The model under review builds one solid part; all positions refer to its coordinate system, in mm. A direction names the side the tool comes from. Round coordinates to 2 decimals unless told otherwise and drop trailing zeros. Loops run counter-clockwise (first coordinate to the right, second up) from the corner with the lowest first, then second, coordinate; pieces in that order, holes last. Notation, with made-up numbers: (-9.75, -24.5) -> (25.25, -24.5) arc R27 cw to (25.25, -4.5) -> close; hole circle Ø5 at (64.25, -29.5). An arc over 180 degrees is marked (long way). Write each question's results on one line, items separated by ' | '. Start each with the question number.
Item 1: For L1, parallel to Y at x = 33, z = -48; L2, parallel to Y at x = 40.5, z = -73; L3, parallel to X at y = 20, z = -83.5, list the stretches that pass through material, from the lowest coordinate up. Write a range as from..to.
Item 2: We need section C-C (z = -68.5). Give the boundary of the cut face in (x, y), and give its area (3 significant figures).
Item 3: Clearance check with flat-ended pins moving along their axes: pin 1 Ø10 at (y, z) = (22, -77.5) entering from +X; pin 2 Ø12 at (x, z) = (39, -17.5) entering from +Y; pin 3 Ø12 at (y, z) = (28.5, -60) entering from +X. State where each tip first meets the part, or that it passes through.
Item 4: We need section D-D (x = 47). Give the boundary of the cut face in (y, z), and give its area (3 significant figures).
Item 5: Tool access review of faces 1 (the cylindrical face through (25.819, 18.961, -50.805)), 2 (the flat face through (26, 0, -44)), 3 (the flat face through (44.45, 19, -80)), 4 (the cylindrical face through (15.322, 31.661, -77.578)), 5 (the flat face through (6.35, 19, -79)): name each direction out of +Z, -Z, +X, -X, +Y, -Y from which nothing blocks a thin tool from reaching the whole face with its end or side.
Item 6: We need section A-A (x = 25.4). Give the boundary of the cut face in (y, z), and give its area (3 significant figures).
Item 7: We need section B-B (y = 28.5). Give the boundary of the cut face in (x, z).
Autodesk Inventor part; units mm, degrees
ref_plane "YZ Plane" through (0, 0, 0) normal (1, 0, 0) x (0, 1, 0)
ref_plane "XZ Plane" through (0, 0, 0) normal (0, 1, 0) x (-1, 0, 0)
ref_plane "XY Plane" through (0, 0, 0) normal (0, 0, 1) x (1, 0, 0)
sketch "Sketch1" plane through (0, 0, 0) normal (0, 1, 0) x (-1, 0, 0)
  line L0 (0, 0) -> (-50.8, 0)
  line L1 (-50.8, 0) -> (-50.8, -88.9)
  line L2 (-50.8, -88.9) -> (0, -88.9)
  line L3 (0, -88.9) -> (0, 0)
  dimension "d0" = 50.8
  dimension "d1" = 88.9
extrude "Extrusion1" add sketch "Sketch1" along normal blind 12.7
sketch "Sketch2" plane through (0, 12.7, 0) normal (0, 1, 0) x (1, 0, 0)
  line L0 (50.8, 0) -> (50.8, 88.9)
  line L1 (50.8, 88.9) -> (0, 88.9)
  line L2 (0, 88.9) -> (0, 0)
  line L3 (6.35, 88.9) -> (44.45, 88.9)
  line L4 (44.45, 88.9) -> (44.45, 69.85)
  line L5 (44.45, 69.85) -> (6.35, 69.85)
  line L6 (6.35, 69.85) -> (6.35, 88.9)
  line L7 (6.35, 79.375) -> (0, 79.375) construction
  line L8 (44.45, 79.375) -> (50.8, 79.375) construction
  circle A0 centre (25.4, 69.85) radius 19.05
  dimension "d4" = 19.05
  dimension "d5" = 6.35
extrude "Extrusion2" add sketch "Sketch2" along normal blind 12.7
sketch "Sketch3" plane through (0, 25.4, 0) normal (0, 1, 0) x (1, 0, 0)
  arc A0 (6.35, 69.85) -> (44.45, 69.85) centre (25.4, 69.85) ccw
  circle A1 centre (25.4, 69.85) radius 12.7
  point P0 (0, 0)
  dimension "d8" = 25.4
extrude "Extrusion3" add sketch "Sketch3" along normal blind 12.7
properties part number "Holes"
Here are the results:
1) L1: y = 0..12.7 | L2: y = 0..25.4 | L3: x = 6.35..44.45
2) outline: (0, 0) -> (50.8, 0) -> (50.8, 12.7) -> (44.4, 12.7) -> (44.4, 25.4) -> (38.03, 25.4) -> (38.03, 38.1) -> (12.77, 38.1) -> (12.77, 25.4) -> (6.4, 25.4) -> (6.4, 12.7) -> (0, 12.7) -> close | area: 1,450 mm2
3) pin 1: stops at x = 44.45 | pin 2: stops at y = 12.7 | pin 3: stops at x = 43.86
4) outline: (0, -88.9) -> (12.7, -88.9) -> (12.7, 0) -> (0, 0) -> close | area: 1,130 mm2
5) face 1: +Z, +Y | face 2: +Z, -Z, +X, -X, -Y | face 3: +Z, -Z, +X, +Y | face 4: +Y | face 5: +Z, -Z, -X, +Y
6) outline: (0, -88.9) -> (25.4, -88.9) -> (25.4, -82.55) -> (38.1, -82.55) -> (38.1, -57.15) -> (25.4, -57.15) -> (25.4, -50.8) -> (12.7, -50.8) -> (12.7, 0) -> (0, 0) -> close | area: 1,940 mm2
7) outline: circle Ø25.4 at (25.4, -69.85)
